from build123d import *

# Parameters (mm, degrees)
SKETCH1_R               = 12.7
BOSS_EXTRUDE1_DEPTH     = 50.8
SKETCH4_R               = 6.35
CUT_EXTRUDE2_DEPTH      = 33.02
CUT_EXTRUDE3_DEPTH      = 54.881536726
CUT_EXTRUDE3_DEPTH_BACK = 54.881536726
SKETCH5_R               = 1.524
CUT_EXTRUDE4_DEPTH      = 15.24
SKETCH7_R               = 1.9939
CUT_EXTRUDE5_DEPTH      = 15.24
SKETCH8_R               = 14.2875
CUT_EXTRUDE6_DEPTH      = 7.62


with BuildPart() as part:
    # Sketch1 → Boss-Extrude1 (new body)
    with BuildSketch(Plane(origin=(0, 0, 0), x_dir=(1, 0, 0), z_dir=(0, 1, 0))):
        with Locations(Location((0, 0, 0), (0, 0, 270))):
            Circle(SKETCH1_R)
    extrude(amount=BOSS_EXTRUDE1_DEPTH)

    # Sketch4 → Cut-Extrude2 (cut)
    with BuildSketch(Plane.XZ):
        with Locations(Location((0, 0, 0), (0, 0, 270))):
            Circle(SKETCH4_R)
    extrude(amount=-CUT_EXTRUDE2_DEPTH, mode=Mode.SUBTRACT)

    # Sketch5 → Cut-Extrude3 (cut, two sides: drawn at the far end of the back side and taken through both)
    with BuildSketch(Plane.XY.offset(-CUT_EXTRUDE3_DEPTH_BACK)):
        with Locations((0, 16.51)):
            Circle(SKETCH5_R)
    extrude(amount=CUT_EXTRUDE3_DEPTH + CUT_EXTRUDE3_DEPTH_BACK, mode=Mode.SUBTRACT)

    # Sketch6 → Cut-Extrude4 (cut)
    with BuildSketch(Plane(origin=(0, 50.8, 0), x_dir=(1, 0, 0), z_dir=(0, 1, 0))):
        with BuildLine():
            Line((-2.238756, 3.467596837), (2.238756, 3.467596837))
            ThreePointArc((2.238756, 3.467596837), (0, -4.1275), (-2.238756, 3.467596837))
        make_face()
    extrude(amount=-CUT_EXTRUDE4_DEPTH, mode=Mode.SUBTRACT)

    # Sketch7 → Cut-Extrude5 (cut)
    with BuildSketch(Plane.XY):
        with Locations(Location((0, 43.18, 0), (0, 0, 90))):
            Circle(SKETCH7_R)
    extrude(amount=-CUT_EXTRUDE5_DEPTH, mode=Mode.SUBTRACT)

    # Sketch8 → Cut-Extrude6 (cut)
    with BuildSketch(Plane.XZ):
        Circle(SKETCH8_R)
    extrude(amount=-CUT_EXTRUDE6_DEPTH, mode=Mode.SUBTRACT)


solid = part.part
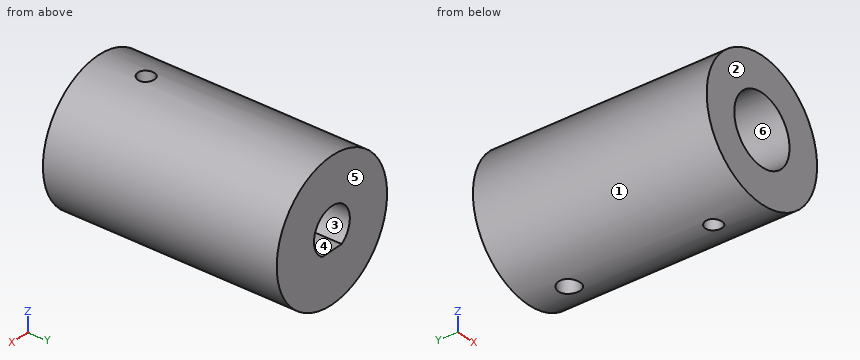
Part model, mm, in its own coordinate system. Face numbers are marked on the shaded views. A direction names the side the tool comes from. Round coordinates to 2 decimals unless told otherwise and drop trailing zeros. Write each loop counter-clockwise with the first axis right and the second up, starting at its lowest first coordinate (ties: lowest second). Pieces come first, ordered by that corner, then holes. Notation, with made-up numbers: M 46,-17.75 L 64,-17.75 A26 cw 64,21.25 Z; hole C 11,18.5 d7. An arc over 180 degrees is marked long. Return JSON: item names as keys, results as strings. Group by question number.
(1) Drill centre lines: probe 1 along Z at (x, y) = (0, 24.5); probe 2 along X at (y, z) = (16.51, -11). Where is each one in solid material? Low to high.
(2) Two-plate mould, pull along Z, no slides. Class the marked faces 1, 2 and 3: +Z half, -Z half, draft (parallel to the pull), parting line (faces both ways), or undercut.
(3) Pin check, flat tips, straight feed: pin 1 Ø6 at (x, z) = (-0.5, 0.5) entering from +Y; pin 2 Ø6 at (x, z) = (-1, 5) entering from -Y; pin 3 Ø4 at (x, z) = (2, -0.5) entering from -Y; pin 4 Ø2.5 at (x, y) = (0, 16.51) entering from +Z. Stop position of each tip, or through.
(4) Saw through at C-C on y = 17. Write the cut outline in (x, z).
(5) Which spindle directions (+Z, -Z, +X, -X, +Y, -Y) get a long thin tool onto all of the face, cutting with end or side? Do the marked faces 4, 5 and 6. Say none if no direction does.
(6) Saw through at A-A on x = 0. Write the cut outline in (y, z).
(7) Saw through at B-B on z = 0. Write the cut outline in (x, y).
Returned:
{
 "1": {"probe 1": "-12.7 to -6.35, 6.35 to 12.7", "probe 2": "-6.35 to -1.52, 1.52 to 6.35"},
 "2": {"face 1": "parting line", "face 2": "draft", "face 3": "undercut"},
 "3": {"pin 1": "y = 35.56", "pin 2": "y = 7.62", "pin 3": "y = 33.02", "pin 4": "through"},
 "4": {"outline": "M -1.44,-12.62 L -1.44,-6.18 A6.35 cw -1.44,6.18 L -1.44,12.62 A12.7 ccw Z; M 1.44,-12.62 A12.7 ccw 1.44,12.62 L 1.44,6.18 A6.35 cw 1.44,-6.18 Z"},
 "5": {"face 4": "+Y", "face 5": "+Z, -Z, +X, -X, +Y", "face 6": "-Y"},
 "6": {"outline": "M 7.62,-12.7 L 14.99,-12.7 L 14.99,-6.35 L 7.62,-6.35 Z; M 7.62,6.35 L 14.99,6.35 L 14.99,12.7 L 7.62,12.7 Z; M 18.03,-12.7 L 41.19,-12.7 L 41.19,-3.47 L 35.56,-3.47 L 35.56,4.13 L 50.8,4.13 L 50.8,12.7 L 18.03,12.7 L 18.03,6.35 L 33.02,6.35 L 33.02,-6.35 L 18.03,-6.35 Z; M 45.17,-12.7 L 50.8,-12.7 L 50.8,-3.47 L 45.17,-3.47 Z"},
 "7": {"outline": "M -12.7,7.62 L -6.35,7.62 L -6.35,33.02 L 6.35,33.02 L 6.35,7.62 L 12.7,7.62 L 12.7,50.8 L 4.13,50.8 L 4.13,35.56 L -4.13,35.56 L -4.13,50.8 L -12.7,50.8 Z"}
}
